```python
from build123d import *

# Parameters (mm, degrees)
SKETCH1_R           = 5
BOSS_EXTRUDE1_DEPTH = 30
CUT_EXTRUDE1_DEPTH  = 10


with BuildPart() as part:
    # Sketch1 → Boss-Extrude1 (new body)
    with BuildSketch(Plane(origin=(0, 0, 0), x_dir=(1, 0, 0), z_dir=(0, 1, 0))):
        Circle(SKETCH1_R)
    extrude(amount=BOSS_EXTRUDE1_DEPTH)

    # Sketch2 → Cut-Extrude1 (cut)
    with BuildSketch(Plane.XZ):
        with BuildLine():
            Line((-2, 3), (2, 3))
            Line((2, 3), (2, 4.582575695))
            ThreePointArc((2, 4.582575695), (0, 5), (-2, 4.582575695))
            Line((-2, 4.582575695), (-2, 3))
        make_face()
    extrude(amount=-CUT_EXTRUDE1_DEPTH, mode=Mode.SUBTRACT)


solid = part.part
```
Verification items for the finished model (mm, model axes). A direction names the side the tool comes from. Coordinates: 2 decimals unless noted, no trailing zeros. Loops run counter-clockwise (first coordinate to the right, second up) from the corner with the lowest first, then second, coordinate; pieces in that order, holes last. Notation, with made-up numbers: (-18, 23.5) - (20, 23.5) arc R25 ccw to (20, 36.5) - close; hole circle Ø6 at (55.25, 73.5). An arc over 180 degrees is marked (long way). Return JSON: item names as keys, results as strings.
1. Section check D-D, the plane x = 3. Record the boundary of the cut face in (y, z), then the cut area to 3 significant figures.
Established:
{"outline": "(0, -4) - (30, -4) - (30, 4) - (0, 4) - close", "area": "240 mm2"}
2. Section check C-C, the plane y = 24.5. Record the boundary of the cut face in (x, z), then the cut area to 3 significant figures.
Established:
{"outline": "circle Ø10 at (0, 0)", "area": "78.5 mm2"}
3. Mould release check, pull along X, two halves, no side actions. Record for faces 3 (the cylindrical face through (3, 15, -4)), 4 (the flat face through (0, 5, 3)), 5 (the flat face through (0, 30, 0)): +X half, -X half, draft (parallel to the pull), parting line (faces both ways), or undercut.
Established:
{"face 3": "parting line", "face 4": "undercut", "face 5": "draft"}
4. Thickness scan on L1, parallel to Y at x = -1, z = 4.5; L2, parallel to X at y = 27, z = -3.75; L3, parallel to X at y = 24.25, z = -0.25. Record the ranges inside material, lowest first.
Established:
{"L1": "y = 10 to 30", "L2": "x = -3.31 to 3.31", "L3": "x = -4.99 to 4.99"}
5. Tool access check on faces 1 (the flat face through (0, 0, 0)), 2 (the flat face through (-2, 5, 4)). Record the directions out of +Z, -Z, +X, -X, +Y, -Y that give a thin tool (end or side, any length) a straight path to the whole face; none if there is none.
Established:
{"face 1": "+Z, -Z, +X, -X, -Y", "face 2": "+Z, -Y"}
6. Go/stop test with flat-tipped pins: pin 1 (6 mm diameter, centred on y = 17.5, z = -3.5, fed in from -X); pin 2 (1 mm diameter, centred on x = 2, y = 17.5, fed in from +Z); pin 3 (1.5 mm diameter, centred on x = -1, y = 5, fed in from +Z). Record where each tip stops, or that it passes through.
Established:
{"pin 1": "stops at x = -4.97", "pin 2": "stops at z = 4.77", "pin 3": "stops at z = 3"}
7. Section check B-B, the plane x = 0. Record the boundary of the cut face in (y, z).
Established:
{"outline": "(0, -5) - (30, -5) - (30, 5) - (10, 5) - (10, 3) - (0, 3) - close"}
8. Section check A-A, the plane z = 4. Record the boundary of the cut face in (x, y).
Established:
{"outline": "(-3, 0) - (-2, 0) - (-2, 10) - (2, 10) - (2, 0) - (3, 0) - (3, 30) - (-3, 30) - close"}
